Verification items for the finished model (mm, model axes). A direction names the side the tool comes from. Give positions to 0.01 mm unless a question says otherwise; leave off trailing zeros. Loops run counter-clockwise (first coordinate to the right, second up) from the corner with the lowest first, then second, coordinate; pieces in that order, holes last. Notation, with made-up numbers: M 44.25,67 L 84.25,67 A15 ccw 84.25,93 Z; hole C 78,-23.75 d8. An arc over 180 degrees is marked long. Answer in a Markdown table with one row per item.
```python
from build123d import *

# Parameters (mm, degrees)
PAD_DEPTH       = 4
SKETCH001_W     = 27
SKETCH001_H     = 19
POCKET_DEPTH    = 1
POCKET001_DEPTH = 27
POCKET002_DEPTH = 27


with BuildPart() as part:
    # Sketch → Pad (new body)
    with BuildSketch(Plane.XY):
        Polygon((-13.5, 9.5), (13.5, 9.5), (13.5, -9.5), (6, -9.5), (6, -12.5), (-6, -12.5), (-6, -9.5), (-13.5, -9.5), align=None)
    extrude(amount=PAD_DEPTH)

    # Sketch001 (on Face9 of Pad) → Pocket (cut)
    with BuildSketch(Plane(origin=(0, 0, 0), x_dir=(1, 0, 0), z_dir=(0, 0, -1))):
        Rectangle(SKETCH001_W, SKETCH001_H)
    extrude(amount=-POCKET_DEPTH, mode=Mode.SUBTRACT)

    # Sketch002 (on Face11 of Pocket) → Pocket001 (cut)
    with BuildSketch(Plane(origin=(-13.5, 0, 0), x_dir=(0, -1, 0), z_dir=(-1, 0, 0))):
        with BuildLine():
            ThreePointArc((12.504744, 1), (11.626065, 3.12132), (9.504744, 4))
            Line((9.504744, 4), (9.504744, 5.572417))
            Line((9.504744, 5.572417), (13.03316, 5.572417))
            Line((13.03316, 5.572417), (13.03316, 1))
            Line((13.03316, 1), (12.504744, 1))
        make_face()
    extrude(amount=-POCKET001_DEPTH, mode=Mode.SUBTRACT)

    # Sketch003 (on Face11 of Pocket001) → Pocket002 (cut)
    with BuildSketch(Plane(origin=(-13.5, 0, 0), x_dir=(0, -1, 0), z_dir=(-1, 0, 0))):
        with BuildLine():
            ThreePointArc((12.001523, 1), (11.26929, 2.767767), (9.501523, 3.5))
            Line((9.501523, 3.5), (9.501523, 1))
            Line((9.501523, 1), (9.324189, 1))
            Line((9.324189, 1), (9.324189, -0.269266))
            Line((9.324189, -0.269266), (10.161053, -0.269266))
            Line((10.161053, -0.269266), (12.001523, -0.269266))
            Line((12.001523, -0.269266), (12.001523, 1))
        make_face()
    extrude(amount=-POCKET002_DEPTH, mode=Mode.SUBTRACT)


solid = part.part
```
Item 1: Sectioned sample at B-B (y = 5.25). Record the cut outline in (x, z).
Reported:
| item | result |
|---|---|
| outline | M -13.5,1 L 13.5,1 L 13.5,4 L -13.5,4 Z |
Item 2: Tool access check on faces 1 (the flat face through (6, -12, 2)), 2 (the flat face through (0, 0, 1)), 3 (the flat face through (0, -9.502, 2)), 4 (the flat face through (-6, -12, 2)). Record the directions out of +Z, -Z, +X, -X, +Y, -Y that give a thin tool (end or side, any length) a straight path to the whole face; none if there is none.
Reported:
| item | result |
|---|---|
| face 1 | +Z, -Z, +X, -Y |
| face 2 | -Z, +X, -X, +Y |
| face 3 | -Z, +X, -X |
| face 4 | +Z, -Z, -X, -Y |
Item 3: Go/stop test with flat-tipped pins: pin 1 (0.5 mm diameter, centred on x = -2, z = 0.5, fed in from +Y); pin 2 (5 mm diameter, centred on x = -9.5, y = -6, fed in from -Z); pin 3 (1.5 mm diameter, centred on x = -6.5, z = 3.5, fed in from -Y). Record where each tip stops, or that it passes through.
Reported:
| item | result |
|---|---|
| pin 1 | stops at y = -12 |
| pin 2 | stops at z = 1 |
| pin 3 | stops at y = -11.79 |
Item 4: Sectioned sample at C-C (x = 9.5). Record the cut outline in (y, z).
Reported:
| item | result |
|---|---|
| outline | M -9.5,1 L 9.5,1 L 9.5,4 L -9.5,4 Z |
Item 5: Scan lines: L1, parallel to Z at x = -3.25, y = -7; L2, parallel to Y at x = 6.5, z = 2.4; L3, parallel to Y at x = 1.5, z = 1.75. Record each from-to range of solid material in increasing order. Write a range as [from, to].
Reported:
| item | result |
|---|---|
| L1 | z = [1, 4] |
| L2 | y = [-9.5, 9.5] |
| L3 | y = [-12.41, -11.89], [-9.5, 9.5] |
Item 6: Release check for a two-part mould opening along Y. For faces 5 (the flat face through (-0.1, -12.002, 0.5)), 6 (the flat face through (10, -9.5, 2)), 7 (the cylindrical face through (0, -11, 3)), 8 (the flat face through (0, 0, 4)) record: released by +Y, released by -Y, zero draft, split by the parting line, or undercut.
Reported:
| item | result |
|---|---|
| face 5 | released by +Y |
| face 6 | released by -Y |
| face 7 | undercut |
| face 8 | zero draft |
